from build123d import *

# Parameters (mm, degrees)
F1_DEPTH = 63.5
F0_W     = 25.4
F0_H     = 19.05
F2_DEPTH = 25.4
F3_DEPTH = 7.9375
F4_R     = 6.35


with BuildPart() as f1:
    # F0 (on Front) → F1 (new body, symmetric)
    with BuildSketch(Plane.XZ):
        Polygon((22.225, 9.525), (-41.275, 9.525), (-41.275, -9.525), (41.275, -9.525), (41.275, 9.525), align=None)
    extrude(amount=F1_DEPTH, both=True)

    # F0 (on Front) → F2 (join, symmetric)
    with BuildSketch(Plane.XZ):
        with BuildLine():
            Line((22.225, 27.0002), (22.225, 9.525))
            Line((22.225, 9.525), (41.275, 9.525))
            Line((41.275, 9.525), (41.275, 27.0002))
            ThreePointArc((41.275, 27.0002), (45.92468, 38.22552), (57.15, 42.8752))
            Line((57.15, 42.8752), (60.325, 42.8752))
            Line((60.325, 42.8752), (60.325, 61.9252))
            Line((60.325, 61.9252), (57.15, 61.9252))
            add(Edge.make_bspline(
                [(54.461055, 61.821533), (55.368857, 61.861839), (56.265521, 61.896322), (57.15, 61.9252)],
                knots=[108.919316, 108.919316, 108.919316, 108.919316, 111.504536, 111.504536, 111.504536, 111.504536], degree=3))
            ThreePointArc((54.461055, 61.821533), (31.521236, 50.72618), (22.225, 27.0002))
        make_face()
        with Locations((73.025, 52.4002)):
            Rectangle(F0_W, F0_H)
    extrude(amount=F2_DEPTH, both=True)

    # F0 (on Front) → F3 (join, symmetric)
    with BuildSketch(Plane.XZ):
        with BuildLine():
            add(Edge.make_bspline(
                [(-41.275, 9.525), (-41.804163, 48.089928), (16.213946, 60.123374), (54.461055, 61.821533)],
                knots=[0, 0, 0, 0, 108.919316, 108.919316, 108.919316, 108.919316], degree=3))
            Line((-41.275, 9.525), (22.225, 9.525))
            Line((22.225, 9.525), (22.225, 27.0002))
            ThreePointArc((22.225, 27.0002), (31.521236, 50.72618), (54.461055, 61.821533))
        make_face()
    extrude(amount=F3_DEPTH, both=True)

    # F4
    f4_edges = [f1.edges().sort_by_distance(p)[0] for p in [
        (-41.275, -63.5, 0),
        (41.275, -63.5, 0),
        (41.275, 63.5, 0),
        (-41.275, 63.5, 0),
    ]]
    fillet(f4_edges, radius=F4_R)

    # F0 (on Front) → F5 (revolve)
    with BuildSketch(Plane.XZ):
        Polygon((60.325, 66.675), (60.325, 61.9252), (85.725, 61.9252), (85.725, 42.8752), (60.325, 42.8752), (60.325, 34.925), (111.125, 34.925), (111.125, 66.675), align=None)
    revolve(axis=Axis((60.325, 0, 50.8), (0, 0, 1)))


solid = f1.part
Here's how the part is built. I have some questions about the finished solid (model axes, mm). A direction names the side the tool comes from. Round coordinates to 2 decimals unless told otherwise and drop trailing zeros. Loops run counter-clockwise (first coordinate to the right, second up) from the corner with the lowest first, then second, coordinate; pieces in that order, holes last. Notation, with made-up numbers: M -30.5,16 L 1.5,16 A22 cw 1.5,41 Z; hole C -21,82 d8. An arc over 180 degrees is marked long. Write each question's results on one line, items separated by ' | '. Start each with the question number.
(1) I want a section at D-D (x = 27). Please give me the cut outline in (y, z) (3 decimals), then the cut area to 3 significant figures.
(2) I want a section at B-B (z = 4). Please give me the cut outline in (x, y) (3 decimals).
(3) On a 3-axis mill with a long thin cutter (end or side, diameter ignored), from which of +Z, -Z, +X, -X, +Y, -Y can I reach the whole of each face in a straight line? I mean faces 1 (the flat face through (-9, -7.938, 28)), 2 (the flat face through (41.275, -1, 4)), 3 (the flat face through (41, -7.938, 59)), 4 (the flat face through (1, 35, 9.525)). Say none if no direction works.
(4) I want a section at A-A (y = 46.5). Please give me the cut outline in (x, z) (3 decimals), then the cut area to 3 significant figures.
(5) Thinking about a two-plate mould opening in Z: for faces 5 (the cylindrical face through (41.8, -0.36, 31.05)), 6 (the cylindrical face through (34.93, 0.51, 60.71)), 7 (the flat face through (60, 1, 66.675)), 8 (the flat face through (-41.275, -1, 0)), which applies, pulls with the +Z half, pulls with the -Z half, needs draft (parallel to the pull), parting line crosses it, or undercut?
(6) Will these pins go through, and if not, where does the flat tip stop? P1, Ø16.5, axis at x = -18, y = -28, coming from the +Z side (3 decimals); P2, Ø8, axis at x = 2.5, z = 34, coming from the +Y side; P3, Ø4, axis at x = 22, z = 40, coming from the -Y side.
(7) I want a section at C-C (y = -32). Please give me the cut outline in (x, z) (3 decimals), then the cut area to 3 significant figures.
(8) If I drill on probe 1 along Z at (x, y) = (41, 44) (3 decimals); probe 2 along Z at (x, y) = (10, 50) (3 decimals); probe 3 along Y at (x, z) = (5.5, 45), over which ranges is the centre line in solid material (lowest first)? Write a range as from..to.
Solved:
1) outline: M -63.5,-9.525 L 63.5,-9.525 L 63.5,9.525 L 25.4,9.525 L 25.4,34.925 L 38.342,34.925 L 38.342,66.675 L -38.342,66.675 L -38.342,34.925 L -25.4,34.925 L -25.4,9.525 L -63.5,9.525 Z | area: 6,140 mm²
2) outline: M -41.275,-57.15 A6.35 ccw -34.925,-63.5 L 34.925,-63.5 A6.35 ccw 41.275,-57.15 L 41.275,57.15 A6.35 ccw 34.925,63.5 L -34.925,63.5 A6.35 ccw -41.275,57.15 Z
3) face 1: -X, -Y | face 2: -Z, +X, +Y, -Y | face 3: none | face 4: -X, +Y
4) outline: M -41.275,-9.525 L 41.275,-9.525 L 41.275,9.525 L -41.275,9.525 Z; M 39.87,34.925 L 80.78,34.925 L 80.78,66.675 L 39.87,66.675 Z | area: 2,870 mm²
5) face 5: pulls with the -Z half | face 6: undercut | face 7: pulls with the +Z half | face 8: needs draft
6) P1: stops at z = 9.525 | P2: stops at y = 7.94 | P3: stops at y = -35.51
7) outline: M -41.275,-9.525 L 41.275,-9.525 L 41.275,9.525 L -41.275,9.525 Z; M 20.871,34.925 L 99.779,34.925 L 99.779,66.675 L 20.871,66.675 Z | area: 4,080 mm²
8) probe 1: z = -9.525..9.525, 34.925..66.675 | probe 2: z = -9.525..9.525 | probe 3: y = -7.94..7.94
